```python
from build123d import *

# Parameters (mm, degrees)
F1_DEPTH = 25


with BuildPart() as f1:
    # F0 (on Top) → F1 (new body)
    with BuildSketch(Plane.XY):
        Polygon((19.639204, -31.020492), (22.021737, 66.735362), (-7.347822, -2.170143), (-14.800628, -18.949018), align=None)
        Polygon((-7.347822, -2.170143), (22.021737, 66.735362), (-52.33696, 57.717394), align=None)
        Polygon((-44.747901, -86.370811), (19.639204, -31.020492), (-14.800628, -18.949018), align=None)
        Polygon((-44.747901, -86.370811), (-14.800628, -18.949018), (-60.489131, -2.934784), align=None)
    extrude(amount=F1_DEPTH)


solid = f1.part
```
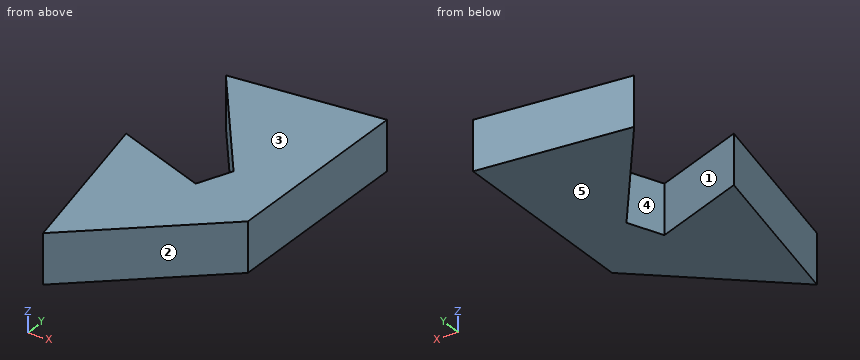
Check sheet for the modelled part. Datum: model origin and axes. Units: mm. Face numbers are marked on the shaded views. A direction names the side the tool comes from. Give positions to 0.01 mm unless a question says otherwise; leave off trailing zeros. Loops run counter-clockwise (first coordinate to the right, second up) from the corner with the lowest first, then second, coordinate; pieces in that order, holes last. Notation, with made-up numbers: M -6.75,18.5 L 30.25,18.5 A13 cw 30.25,34.5 Z; hole C -18,-32 d6. An arc over 180 degrees is marked long. Answer in a Markdown table with one row per item.
1) Cross-section at C-C (x = -49). Enter the section's corners in (y, z).
Solutions:
| item | result |
|---|---|
| outline | M -63.83,0 L -6.96,0 L -6.96,25 L -63.83,25 Z; M 53.28,0 L 58.12,0 L 58.12,25 L 53.28,25 Z |
2) Cross-section at B-B (z = 16.5). Enter the section's corners in (x, y), plus the area to 3 significant figures.
Solutions:
| item | result |
|---|---|
| outline | M -60.49,-2.93 L -44.75,-86.37 L 19.64,-31.02 L 22.02,66.74 L -52.34,57.72 L -7.35,-2.17 L -14.8,-18.95 Z |
| area | 7,240 mm^2 |
3) Cross-section at D-D (y = 45.5). Enter the section's corners in (x, z), plus the area to 3 significant figures.
Solutions:
| item | result |
|---|---|
| outline | M -43.16,0 L 21.5,0 L 21.5,25 L -43.16,25 Z |
| area | 1,620 mm^2 |
4) Mould release check, pull along X, two halves, no side actions. Record for the marked faces 1, 2 and 3: released by +X, released by -X, zero draft, split by the parting line, or undercut.
Solutions:
| item | result |
|---|---|
| face 1 | undercut |
| face 2 | released by +X |
| face 3 | zero draft |
5) Thickness scan on line 1 (Y direction, x = -13.5, z = 17.5); line 2 (X direction, y = 7, z = 17.25); line 3 (X direction, y = 8, z = 12.75). Record the ranges inside material, lowest first.
Solutions:
| item | result |
|---|---|
| line 1 | y = -59.51 to -16.02, 6.02 to 62.43 |
| line 2 | x = -14.24 to 20.57 |
| line 3 | x = -14.99 to 20.59 |
6) Tool access check on the marked faces 4 and 5. Record the directions out of +Z, -Z, +X, -X, +Y, -Y that give a thin tool (end or side, any length) a straight path to the whole face; none if there is none.
Solutions:
| item | result |
|---|---|
| face 4 | +Z, -Z |
| face 5 | -Z, +X, -X, +Y, -Y |
7) Cross-section at A-A (x = -30). Enter the section's corners in (y, z).
Solutions:
| item | result |
|---|---|
| outline | M -73.69,0 L -13.62,0 L -13.62,25 L -73.69,25 Z; M 27.98,0 L 60.43,0 L 60.43,25 L 27.98,25 Z |
8) Depth check by flat-ended pin: pin 1 (5 mm diameter, centred on x = -9.5, z = 15.5, fed in from +Y); pin 2 (6 mm diameter, centred on x = -16, z = 7.5, fed in from -Y); pin 3 (6 mm diameter, centred on x = -41, z = 19.5, fed in from -Y). Enter the tip coordinate at first touch or a pass-through.
Solutions:
| item | result |
|---|---|
| pin 1 | stops at y = 63.22 |
| pin 2 | stops at y = -64.24 |
| pin 3 | stops at y = -85.73 |
